from build123d import *

# Parameters (mm, degrees)
SKETCH_2_R          = 1.5
EXTRUDE_1_DEPTH     = 4
SKETCH_3_R          = 3
EXTRUDE_2_DEPTH     = 1
FILLET_1_R          = 0.5
CUT_EXTRUDE_2_DEPTH = 0.5
CHAMFER_1_SIZE      = 0.3


with BuildPart() as part:
    # 草图2 → 凸台-拉伸1 (new body)
    with BuildSketch(Plane(origin=(0, 0, 0), x_dir=(1, 0, 0), z_dir=(0, 1, 0))):
        with Locations(Location((0, 0, 0), (0, 0, 270))):
            Circle(SKETCH_2_R)
    extrude(amount=EXTRUDE_1_DEPTH)

    # 草图3 → 凸台-拉伸2 (add)
    with BuildSketch(Plane.XZ):
        with Locations(Location((0, 0, 0), (0, 0, 270))):
            Circle(SKETCH_3_R)
    extrude(amount=EXTRUDE_2_DEPTH)

    # 圆角1
    fillet_1_edges = [part.edges().sort_by_distance(p)[0] for p in [
        (0, 0, 3),
        (0, -1, 3),
    ]]
    fillet(fillet_1_edges, radius=FILLET_1_R - 0.0001)  # a hair under: the kernel refuses the full size

    # 草图4 → 切除-拉伸2 (cut)
    with BuildSketch(Plane.XZ.offset(1)):
        Polygon((-1.5, -0.2), (-0.2, -0.2), (-0.2, -1.5), (0.2, -1.5), (0.2, -0.2), (1.5, -0.2), (1.5, 0.2), (0.2, 0.2), (0.2, 1.5), (-0.2, 1.5), (-0.2, 0.2), (-1.5, 0.2), align=None)
    extrude(amount=-CUT_EXTRUDE_2_DEPTH, mode=Mode.SUBTRACT)

    # 倒角1
    chamfer_1_edges = [part.edges().sort_by_distance(p)[0] for p in [
        (0, 4, -1.5),
    ]]
    chamfer(chamfer_1_edges, length=CHAMFER_1_SIZE)


solid = part.part
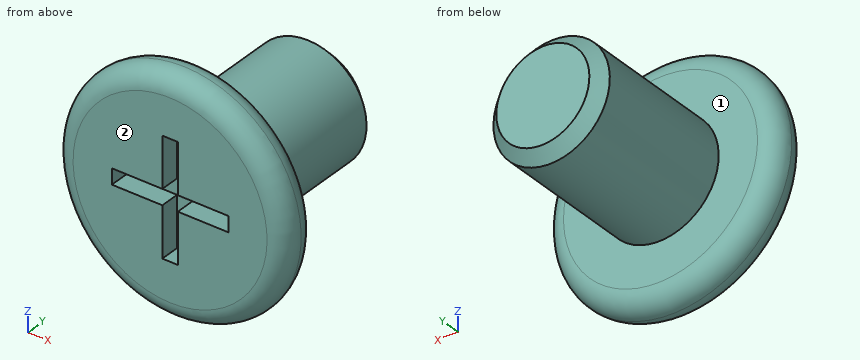
Work out the finished part from the listing and answer in its coordinate system (mm). Face numbers are marked on the shaded views. A direction names the side the tool comes from. Round coordinates to 2 decimals unless told otherwise and drop trailing zeros. Write each loop counter-clockwise with the first axis right and the second up, starting at its lowest first coordinate (ties: lowest second). Pieces come first, ordered by that corner, then holes.
1) A cutting plane is placed at D-D (y = 2.1). Give the vertices of the cut face in (x, z), plus the area to 3 significant figures.
2) Straight lines are drawn through the part: line 1 (Y direction, x = -0.95, z = 1.5); line 2 (X direction, y = 2.85, z = 0). For each, find the intervals that lie inside material, in ascending order.
3) A tool of negligible diameter and unlimited length cuts with its end or side. For the marked faces 1 and 2, from which of +Z, -Z, +X, -X, +Y, -Y can it reach the whole face along a straight path? Write none if from no direction.
4) A cutting plane is placed at C-C (y = -0.6). Give the vertices of the cut face in (x, z).
5) Given pin 1 Ø0.6 at (x, y) = (-1, -0.5) entering from -Z; pin 2 Ø3 at (x, y) = (0.5, 2) entering from +Z; pin 3 Ø1.5 at (y, z) = (1.5, 2.5) entering from +X; pin 4 Ø0.6 at (y, z) = (-0.5, 0.5) entering from +X, each flat-ended and moving along its own axis, determine where each tip first touches the part or whether it passes through.
Completed:
1. outline: circle Ø3 at (0, 0)
1. area: 7.07 mm2
2. line 1: y = -1 to 0
2. line 2: x = -1.5 to 1.5
3. face 1: +Y
3. face 2: +Z, -Z, +X, -X, -Y
4. outline: circle Ø5.98 at (0, 0); hole (-1.5, -0.2) - (-0.2, -0.2) - (-0.2, -1.5) - (0.2, -1.5) - (0.2, -0.2) - (1.5, -0.2) - (1.5, 0.2) - (0.2, 0.2) - (0.2, 1.5) - (-0.2, 1.5) - (-0.2, 0.2) - (-1.5, 0.2) - close
5. pin 1: stops at z = -2.92
5. pin 2: stops at z = 1.5
5. pin 3: passes through
5. pin 4: stops at x = 2.99
